Here's how the part is built. I have some questions about the finished solid (model axes, mm). A direction names the side the tool comes from. Coordinates: 2 decimals unless noted, no trailing zeros. Write each loop counter-clockwise with the first axis right and the second up, starting at its lowest first coordinate (ties: lowest second). Pieces come first, ordered by that corner, then holes. Notation, with made-up numbers: M 50.25,10 L 59.25,10 A13 cw 59.25,31 Z; hole C -1.5,63 d9. An arc over 180 degrees is marked long. Use one line per item in the form item = value. Start each with the question number.
1. I want a section at B-B, the plane x = 18.5. List the corners of the cut face in (y, z) for me (3 decimals).
2. Thinking about a two-plate mould opening in Z: for faces 1 (the face through (16, -17, 6.35)), 2 (the face through (8.26, -17.22, 8.16)), 3 (the face through (0, -17, 32)), which applies, released by +Z, released by -Z, zero draft, split by the parting line, or undercut?
3. On a 3-axis mill with a long thin cutter (end or side, diameter ignored), from which of +Z, -Z, +X, -X, +Y, -Y can I reach the whole of each face in a straight line? I mean faces 4 (the face through (32, -17, 6.35)), 5 (the face through (6.35, -17, 35)), 6 (the face through (19, -17, 0)). Say none if no direction works.
4. I'm going to push flat-ended pins straight in: pin 1 Ø6 at (x, z) = (10, 56.5) entering from -Y; pin 2 Ø7.5 at (x, y) = (14.5, -13.5) entering from +Z; pin 3 Ø10.5 at (x, y) = (32.5, -17) entering from +Z; pin 4 Ø10.5 at (y, z) = (-14.5, 27.5) entering from +X. Where does each tip first touch, or does it pass through?
5. I want a section at C-C, the plane z = 49.5. List the corners of the cut face in (x, y) for me (3 decimals).
6. Please list where this line runs through material, in increasing order: line 1 along X through (y, z) = (-4, 29). Write a range as [from, to].
from build123d import *

# Parameters (mm, degrees)
F1_DEPTH = 34.925
F2_R     = 3.175
F3_DEPTH = 34.925


with BuildPart() as f1:
    # F0 (on Front) → F1 (new body)
    with BuildSketch(Plane.XZ):
        with BuildLine():
            Line((3.175, 63.5), (0, 63.5))
            Line((0, 63.5), (0, 0))
            Line((0, 0), (38.1, 0))
            Line((38.1, 0), (38.1, 6.35))
            Line((38.1, 6.35), (12.7, 6.35))
            ThreePointArc((12.7, 6.35), (8.209872, 8.209872), (6.35, 12.7))
            Line((6.35, 12.7), (6.35, 60.325))
            ThreePointArc((6.35, 60.325), (5.420064, 62.570064), (3.175, 63.5))
        make_face()
    extrude(amount=F1_DEPTH)

    # F2 (on face) → F3 (join, through all)
    with BuildSketch(Plane.XZ.offset(34.925)):
        with Locations((4.7625, 60.325)):
            Circle(F2_R)
        with Locations((22.225, 4.7625)):
            Circle(F2_R)
    extrude(amount=-F3_DEPTH)


solid = f1.part
Answer list:
q1.outline = M -34.925,0 L 0,0 L 0,6.35 L -34.925,6.35 Z
q2.face_1 = released by +Z
q2.face_2 = undercut
q2.face_3 = zero draft
q3.face_4 = +Z, +X, +Y, -Y
q3.face_5 = +X, +Y, -Y
q3.face_6 = -Z, +X, -X, +Y, -Y
q4.pin_1 = through
q4.pin_2 = 6.66
q4.pin_3 = 6.35
q4.pin_4 = 6.35
q5.outline = M 0,-34.925 L 6.35,-34.925 L 6.35,0 L 0,0 Z
q6.line_1 = [0, 6.35]
